Source: CAD feature listing. Evaluate the final solid. Frame: model axes, mm. Face numbers are marked on the shaded views. Give positions to 0.01 mm unless a question says otherwise; leave off trailing zeros. Order: outer loops, then holes, each group sorted by start corner. A loop starts at its lowest first (then second) coordinate and runs counter-clockwise, first axis right, second up. Notation, with made-up numbers: M 76,-31.75 L 108,-31.75 A3 cw 108,-27.75 Z; hole C 54.5,72.25 d1. An arc over 180 degrees is marked long. Use CSV: the item, a comma, the result in double quotes. Start each with the question number.
1. Section query A-A, the plane y = -1.1. Return the cut outline in (x, z).
2. Line query: line 1 along Z through (x, y) = (0, -0.9); line 2 along Z through (x, y) = (0, -0.1); line 3 along X through (y, z) = (-1.5, 1). Output: solid intervals per line, ascending. Write a range as [from, to].
3. Mould query, pull axis X, two halves, no side actions, for the marked faces 1, 2 and 3. Classes: released by +X, released by -X, zero draft, split by the parting line, or undercut.
4. Pin query (flat end, axial travel): P1, Ø3, axis at x = -2.5, z = -3.5, coming from the +Y side (3 decimals); P2, Ø1, axis at x = 1.5, y = -1, coming from the -Z side; P3, Ø3.5, axis at x = 0, z = 0, coming from the +Y side; P4, Ø1, axis at x = -3.5, y = 0.5, coming from the +Z side. Return the tip coordinate at first contact, or that it passes through.
5. Section query B-B, the plane y = 1.05. Return the cut outline in (x, z), plus the area to 3 significant figures.
from build123d import *


with BuildPart() as part:
    # Sketch3 → Revolve1 (revolve)
    with BuildSketch(Plane.XY):
        with BuildLine():
            Line((-2, 1.765), (-2, -1.765))
            Line((-2, -1.765), (-3.3229, -1.765))
            Line((-3.3229, -1.765), (-3.3229, -1.65025))
            Line((-3.3229, -1.65025), (-3.43, -1.54315))
            Line((-3.43, -1.54315), (-3.43, -0.628975))
            Line((-3.43, -0.628975), (-3.3229, -0.521875))
            Line((-3.3229, -0.521875), (-3.307578125, -0.521875))
            ThreePointArc((-3.307578125, -0.521875), (-3.231508903, -0.490366097), (-3.2, -0.414296875))
            Line((-3.2, -0.414296875), (-3.2, -0.342578125))
            ThreePointArc((-3.2, -0.342578125), (-3.231508903, -0.266508903), (-3.307578125, -0.235))
            Line((-3.307578125, -0.235), (-4.2325, -0.235))
            ThreePointArc((-4.2325, -0.235), (-4.329727182, -0.194727182), (-4.37, -0.0975))
            Line((-4.37, -0.0975), (-4.37, 0.04))
            Line((-4.37, 0.04), (-4.2325, 0.04))
            Line((-4.2325, 0.04), (-4.2325, 0.1775))
            Line((-4.2325, 0.1775), (-4.37, 0.1775))
            Line((-4.37, 0.1775), (-4.37, 0.315))
            Line((-4.37, 0.315), (-4.2325, 0.315))
            Line((-4.2325, 0.315), (-4.2325, 0.4525))
            Line((-4.2325, 0.4525), (-4.37, 0.4525))
            Line((-4.37, 0.4525), (-4.37, 1.6579))
            Line((-4.37, 1.6579), (-4.2629, 1.765))
            Line((-4.2629, 1.765), (-2, 1.765))
        make_face()
    revolve(axis=Axis((0, -1.765, 0), (0, 1, 0)))


solid = part.part
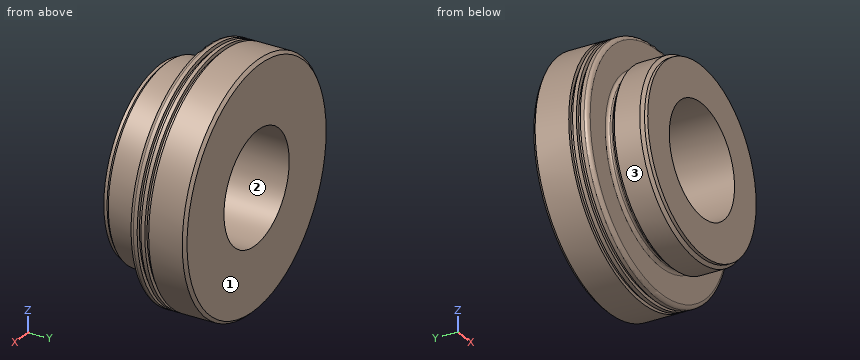
Result set:
1,outline,"C 0,0 d6.86; hole C 0,0 d4"
2,line 1,"[-3.43, -2], [2, 3.43]"
2,line 2,"[-4.37, -2], [2, 4.37]"
2,line 3,"[-3.28, -1.73], [1.73, 3.28]"
3,face 1,"zero draft"
3,face 2,"undercut"
3,face 3,"split by the parting line"
4,P1,"y = 1.765"
4,P2,"z = -3.28"
4,P3,"through"
4,P4,"z = 3.18"
5,outline,"C 0,0 d8.74; hole C 0,0 d4"
5,area,"47.4 mm2"
